Autodesk Inventor part; units mm, degrees
ref_plane "Work Plane1" through (-9.2786, -9.2786, 2.6) normal (0, 0, -1) x (0, 1, 0)
ref_plane "YZ Plane" through (0, 0, 0) normal (1, 0, 0) x (0, 1, 0)
ref_plane "XZ Plane" through (0, 0, 0) normal (0, 1, 0) x (-1, 0, 0)
sketch "Sketch1" plane through (0, 0, 0) normal (0, 0, 1) x (1, 0, 0)
  line L0 (3.9818, -0.3812) -> (1.7924, -3.5759)
  arc A0 (1.6608, -3.6389) -> (1.7924, -3.5759) centre (0, 0) ccw
  line L1 (1.6608, -3.6389) -> (-2.2007, -3.3402)
  arc A1 (-2.321, -3.2577) -> (-2.2007, -3.3402) centre (0, 0) ccw
  line L2 (-2.321, -3.2577) -> (-3.993, 0.2357)
  arc A2 (-3.9818, 0.3812) -> (-3.993, 0.2357) centre (0, 0) ccw
  line L3 (-3.9818, 0.3812) -> (-1.7924, 3.5759)
  arc A3 (-1.6608, 3.6389) -> (-1.7924, 3.5759) centre (0, 0) ccw
  line L4 (-1.6608, 3.6389) -> (2.2007, 3.3402)
  arc A4 (2.321, 3.2577) -> (2.2007, 3.3402) centre (0, 0) ccw
  line L5 (2.321, 3.2577) -> (3.993, -0.2357)
  arc A5 (3.9818, -0.3812) -> (3.993, -0.2357) centre (0, 0) ccw
  circle A6 centre (0, 0) radius 5
  point P0 (0, 0)
  dimension "d0" = 10
ref_plane "Work Plane1" through (-9.2786, -9.2786, 2.6) normal (0, 0, -1) x (0, 1, 0)
extrude "Extrusion1" add sketch "Sketch1" along normal up to surface (2.6 mm away)
properties part number "Power_Transmission_Spacer_One"
The listing builds one solid part. Answer for the finished solid, in the listing's coordinates (mm). A direction names the side the tool comes from. Coordinates: 2 decimals unless noted, no trailing zeros. Order: outer loops, then holes, each group sorted by start corner. A loop starts at its lowest first (then second) coordinate and runs counter-clockwise, first axis right, second up. Notation, with made-up numbers: (70, 10) -> (96, 10) arc R30 ccw to (96, 44) -> close; hole circle Ø9 at (5.25, -19.75). An arc over 180 degrees is marked (long way). Answer in a Markdown table with one row per item. Add a question column.
Item 1: Find section A-A (x = -3.25). Write down the section's boundary in (y, z).
Item 2: Find section C-C (z = 1.8). Write down the section's boundary in (x, y).
Item 3: Find the intervals of material crossed by L1, parallel to X at y = 0.75, z = 1.4; L2, parallel to Y at x = -3.5, z = 2.45; L3, parallel to X at y = -3, z = 1.9, in increasing order. Write a range as from..to.
Item 4: Find section B-B (y = 2). Write down the section's boundary in (x, z).
Item 5: Which of the six approach directions +Z, -Z, +X, -X, +Y, -Y give full straight-line access (tool end or side, diameter ignored) to faces 1 (the face through (-3, 3, 0)), 2 (the face through (2.9, -1.96, 1.28))?
Result set:
| question | item | result |
|---|---|---|
| 1 | outline | (-3.8, 0) -> (-1.32, 0) -> (-1.32, 2.6) -> (-3.8, 2.6) -> close; (1.45, 0) -> (3.8, 0) -> (3.8, 2.6) -> (1.45, 2.6) -> close |
| 2 | outline | circle Ø10 at (0, 0); hole (-3.99, 0.24) -> (-2.32, -3.26) arc R4.14 ccw to (-2.2, -3.34) -> (1.66, -3.64) arc R3.97 ccw to (1.79, -3.58) -> (3.98, -0.38) arc R3.84 ccw to (3.99, -0.24) -> (2.32, 3.26) arc R4.14 ccw to (2.2, 3.34) -> (-1.66, 3.64) arc R3.97 ccw to (-1.79, 3.58) -> (-3.98, 0.38) arc R3.84 ccw to start |
| 3 | L1 | x = -4.94..-3.73, 3.52..4.94 |
| 3 | L2 | y = -3.57..-0.79, 1.08..3.57 |
| 3 | L3 | x = -4..-2.44, 2.19..4 |
| 4 | outline | (-4.58, 0) -> (-2.87, 0) -> (-2.87, 2.6) -> (-4.58, 2.6) -> close; (2.92, 0) -> (4.58, 0) -> (4.58, 2.6) -> (2.92, 2.6) -> close |
| 5 | face 1 | -Z, +X, -X, +Y, -Y |
| 5 | face 2 | +Z, -Z |
